The listing builds one solid part. Answer for the finished solid, in the listing's coordinates (mm). A direction names the side the tool comes from. Round coordinates to 2 decimals unless told otherwise and drop trailing zeros. Write each loop counter-clockwise with the first axis right and the second up, starting at its lowest first coordinate (ties: lowest second). Pieces come first, ordered by that corner, then holes. Notation, with made-up numbers: (41, -11) - (69, -11) arc R23 ccw to (69, 4) - close; hole circle Ø6 at (25, 70). An arc over 180 degrees is marked (long way). Return JSON: item names as keys, results as strings. Group by question number.
(1) Find the intervals of material crossed by line 1 along X through (y, z) = (-9.5, 0.95); line 2 along Y through (x, z) = (-21.56, 1.25); line 3 along Y through (x, z) = (-1, 0.75) (3 decimals), in increasing order. Write a range as [from, to].
(2) Section B-B, the plane y = -3 is taken. Write down the section's boundary in (x, z), then the cut area to 3 significant figures.
(3) Each of these flat-tipped pins is pushed along its axis until it touches: pin 1 (1.5 mm diameter, centred on y = -21.5, z = 1.5, fed in from +X); pin 2 (3 mm diameter, centred on x = 13.5, y = 6.5, fed in from -Z); pin 3 (1 mm diameter, centred on x = 3, y = -18, fed in from -Z); pin 4 (0.9 mm diameter, centred on x = -5, z = 1.5, fed in from -Y). Where does it stop, or does it pass through?
(4) Determine the mould class of faces 1 (the cylindrical face through (-22.56, 9.39, 1.48)), 2 (the flat face through (-25, -21, 1)), 3 (the cylindrical face through (5.154, 7.249, 1.479)), 4 (the flat face through (20, -23, 1)) for opening direction Y: +Y half, -Y half, draft (parallel to the pull), parting line (faces both ways), or undercut.
(5) Which of the six approach directions +Z, -Z, +X, -X, +Y, -Y give full straight-line access (tool end or side, diameter ignored) to faces 5 (the flat face through (35, -14, 1)), 6 (the flat face through (-37, -7.014, 1)), 7 (the flat face through (37, 2.986, 1)), 8 (the flat face through (-35, 12, 1)), 9 (the flat face through (0, -20, 1))?
(6) Section C-C, the plane y = 7.2 is taken. Write down the section's boundary in (x, z) (3 decimals).
(7) Section A-A, the plane x = -13 is taken. Write down the section's boundary in (y, z).
(8) Section D-D, the plane z = 0.65 is taken. Give the number of separate pieces and of enclosed holes in the cut face, then the cut area to 3 significant figures.
```python
from build123d import *

# Parameters (mm, degrees)
SKETCH_1_R      = 8
SKETCH_1_R_2    = 1
EXTRUDE_1_DEPTH = 3


with BuildPart() as part:
    # 草图1 → 凸台-拉伸1 (new body)
    with BuildSketch(Plane.XY):
        Polygon((-35, -7.01394437), (-35, -20), (-25, -20), (-25, -23), (-15, -23), (-15, -20), (15, -20), (15, -23), (25, -23), (25, -20), (35, -20), (35, -7.01394437), (38, -7.01394437), (38, 2.98605563), (35, 2.98605563), (35, 20), (25, 20), (25, 23), (15, 23), (15, 20), (-15, 20), (-15, 23), (-25, 23), (-25, 20), (-35, 20), (-35, 2.98605563), (-38, 2.98605563), (-38, -7.01394437), align=None)
        with Locations((-13, 1.171567705)):
            Circle(SKETCH_1_R, mode=Mode.SUBTRACT)
        with Locations(Location((13, 1.171567705, 0), (0, 0, 180))):
            Circle(SKETCH_1_R, mode=Mode.SUBTRACT)
        with Locations((-21.56, 9.341567705)):
            Circle(SKETCH_1_R_2, mode=Mode.SUBTRACT)
        with Locations(Location((-21.56, -9.341567705, 0), (0, 0, 180))):
            Circle(SKETCH_1_R_2, mode=Mode.SUBTRACT)
        with Locations((21.56, -9.341567705)):
            Circle(SKETCH_1_R_2, mode=Mode.SUBTRACT)
        with Locations(Location((21.56, 9.341567705, 0), (0, 0, 180))):
            Circle(SKETCH_1_R_2, mode=Mode.SUBTRACT)
        with BuildLine():
            Line((-2.93, 9.425), (2.93, 9.425))
            ThreePointArc((2.93, 9.425), (5.155, 7.2), (2.93, 4.975))
            Line((2.93, 4.975), (-2.93, 4.975))
            ThreePointArc((-2.93, 4.975), (-5.155, 7.2), (-2.93, 9.425))
        make_face(mode=Mode.SUBTRACT)
    extrude(amount=EXTRUDE_1_DEPTH)


solid = part.part
```
Working result:
{
 "1": {"line 1": "x = [-35, -22.55], [-20.57, 20.57], [22.55, 35]", "line 2": "y = [-23, -10.34], [-8.34, 8.34], [10.34, 23]", "line 3": "y = [-20, 4.975], [9.425, 20]"},
 "2": {"outline": "(-38, 0) - (-19.83, 0) - (-19.83, 3) - (-38, 3) - close; (-6.17, 0) - (6.17, 0) - (6.17, 3) - (-6.17, 3) - close; (19.83, 0) - (38, 0) - (38, 3) - (19.83, 3) - close", "area": "146 mm^2"},
 "3": {"pin 1": "stops at x = 25", "pin 2": "passes through", "pin 3": "stops at z = 0", "pin 4": "stops at y = -20"},
 "4": {"face 1": "undercut", "face 2": "draft", "face 3": "undercut", "face 4": "-Y half"},
 "5": {"face 5": "+Z, -Z, +X, -Y", "face 6": "+Z, -Z, -X, -Y", "face 7": "+Z, -Z, +X, +Y", "face 8": "+Z, -Z, -X, +Y", "face 9": "+Z, -Z, -Y"},
 "6": {"outline": "(-35, 0) - (-18.259, 0) - (-18.259, 3) - (-35, 3) - close; (-7.741, 0) - (-5.155, 0) - (-5.155, 3) - (-7.741, 3) - close; (5.155, 0) - (7.741, 0) - (7.741, 3) - (5.155, 3) - close; (18.259, 0) - (35, 0) - (35, 3) - (18.259, 3) - close"},
 "7": {"outline": "(-20, 0) - (-6.83, 0) - (-6.83, 3) - (-20, 3) - close; (9.17, 0) - (20, 0) - (20, 3) - (9.17, 3) - close"},
 "8": {"separate pieces": "1", "enclosed holes": "7", "area": "2,520 mm^2"}
}
